```python
from build123d import *

# Parameters (mm, degrees)
SKETCH1_W               = 52
SKETCH1_H               = 46
SKETCH1_R               = 1.15
SKETCH1_R_2             = 11.5
SKETCH1_W_2             = 4.3
SKETCH1_H_2             = 18
BOSS_EXTRUDE1_DEPTH     = 4
BOSS_EXTRUDE2_DEPTH     = 4
BOSS_EXTRUDE3_DEPTH     = 44
CHAMFER1_SIZE           = 25
CUT_EXTRUDE1_DEPTH      = 70.491006612
CUT_EXTRUDE1_DEPTH_BACK = 70.491006612
SKETCH4_R               = 1.15
FILLET1_R               = 5
FILLET2_R               = 1


with BuildPart() as part:
    # Sketch1 → Boss-Extrude1 (new body)
    # profile 1 of 4: a face of its own
    with BuildSketch(Plane.XY):
        with Locations((0, -2)):
            Rectangle(SKETCH1_W, SKETCH1_H)
        with Locations((15.5, 15.5)):
            Circle(SKETCH1_R, mode=Mode.SUBTRACT)
        with Locations((15.5, -15.5)):
            Circle(SKETCH1_R, mode=Mode.SUBTRACT)
        with Locations((-15.5, -15.5)):
            Circle(SKETCH1_R, mode=Mode.SUBTRACT)
        with Locations((-15.5, 15.5)):
            Circle(SKETCH1_R, mode=Mode.SUBTRACT)
        Circle(SKETCH1_R_2, mode=Mode.SUBTRACT)
    # profile 2 of 4: a face of its own
    with BuildSketch(Plane.XY):
        with Locations((-13.488188518, -34)):
            Rectangle(SKETCH1_W_2, SKETCH1_H_2)
    # profile 3 of 4: a face of its own
    with BuildSketch(Plane.XY):
        with Locations((13.488188518, -34)):
            Rectangle(SKETCH1_W_2, SKETCH1_H_2)
    # profile 4 of 4: a face of its own
    with BuildSketch(Plane.XY):
        Polygon((3.5, -26), (4.5, -25), (-4.5, -25), (-3.5, -26), align=None)
    extrude(amount=BOSS_EXTRUDE1_DEPTH)

    # Sketch2 → Boss-Extrude2 (add)
    with BuildSketch(Plane.XY):
        Polygon((26, 21), (22, 21), (22, -17), (18, -21), (-18, -21), (-22, -17), (-22, 21), (-26, 21), (-26, -25), (-15.638188518, -25), (-15.638188518, -43), (-11.338188518, -43), (-11.338188518, -25), (-4.5, -25), (-3.5, -26), (3.5, -26), (4.5, -25), (11.338188518, -25), (11.338188518, -43), (15.638188518, -43), (15.638188518, -25), (26, -25), align=None)
    extrude(amount=-BOSS_EXTRUDE2_DEPTH)

    # Sketch3 → Boss-Extrude3 (add)
    with BuildSketch(Plane(origin=(0, 0, -4), x_dir=(-1, 0, 0), z_dir=(0, 0, -1))):
        Polygon((-26, -25), (-26, -17), (-22, -17), (-18, -21), (18, -21), (22, -17), (26, -17), (26, -25), (15.638188518, -25), (15.638188518, -43), (11.338188518, -43), (11.338188518, -25), (4.5, -25), (3.5, -26), (-3.5, -26), (-4.5, -25), (-11.338188518, -25), (-11.338188518, -43), (-15.638188518, -43), (-15.638188518, -25), align=None)
    extrude(amount=BOSS_EXTRUDE3_DEPTH)

    # Chamfer1
    chamfer1_edges = [part.edges().sort_by_distance(p)[0] for p in [
        (-24, -17, -4),
        (24, -17, -4),
    ]]
    chamfer(chamfer1_edges, length=CHAMFER1_SIZE)

    # Sketch4 → Cut-Extrude1 (cut, two sides: drawn at the far end of the back side and taken through both)
    with BuildSketch(Plane(origin=(0, 0, 0), x_dir=(0, 0, -1), z_dir=(1, 0, 0)).offset(-CUT_EXTRUDE1_DEPTH_BACK)):
        with Locations(Location((34, -35, 0), (0, 0, 270))):
            Circle(SKETCH4_R)
        with Locations(Location((12, -35, 0), (0, 0, 270))):
            Circle(SKETCH4_R)
    extrude(amount=CUT_EXTRUDE1_DEPTH + CUT_EXTRUDE1_DEPTH_BACK, mode=Mode.SUBTRACT)

    # Fillet1
    fillet1_edges = [part.edges().sort_by_distance(p)[0] for p in [
        (15.638188518, -25, -22),
        (-15.638188518, -25, -22),
    ]]
    fillet(fillet1_edges, radius=FILLET1_R)

    # Fillet2
    # the kernel refuses this fillet: 1 mm, written as the material it adds along each edge
    with BuildSketch(Plane(origin=(-22, -17, -29), x_dir=(0, 0.7071067811865475, 0.7071067811865475), z_dir=(-1, 0, 0))) as fillet2_piece_1_section:
        with BuildLine():
            CenterArc((FILLET2_R * 0.414213562373, FILLET2_R), FILLET2_R, 225, 45)
            Line((-FILLET2_R * 0.292893218813, FILLET2_R * 0.292893218813), (0, 0))
            Line((0, 0), (FILLET2_R * 0.414213562373, 0))
        make_face()
    fillet2_piece_1 = extrude(amount=4, mode=Mode.PRIVATE)
    fillet2_piece_1 = split(fillet2_piece_1, bisect_by=Plane(origin=(-22.109509858, -16.890490142, -28.87205582), z_dir=(0.7071067811865658, 0.7071067811865294, 0)), keep=Keep.TOP, mode=Mode.PRIVATE)
    add(fillet2_piece_1)
    with BuildSketch(Plane(origin=(-22, -17, -29), x_dir=(0, 0.7071067811865475, 0.7071067811865475), z_dir=(-1, 0, 0))) as fillet2_piece_2_section:
        with BuildLine():
            CenterArc((FILLET2_R * 0.414213562373, FILLET2_R), FILLET2_R, 225, 45)
            Line((-FILLET2_R * 0.292893218813, FILLET2_R * 0.292893218813), (0, 0))
            Line((0, 0), (FILLET2_R * 0.414213562373, 0))
        make_face()
    fillet2_piece_2 = extrude(amount=4, mode=Mode.PRIVATE)
    fillet2_piece_2 = split(fillet2_piece_2, bisect_by=Plane(origin=(-23.045900005, -15.954099995, -29.028101444), z_dir=(-0.7071067811865658, -0.7071067811865294, 0)), keep=Keep.TOP, mode=Mode.PRIVATE)
    add(fillet2_piece_2)
    with BuildSketch(Plane(origin=(-22, 8, -4), x_dir=(0, 1, 0), z_dir=(-1, 0, 0))) as fillet2_piece_3:
        with BuildLine():
            CenterArc((FILLET2_R * 0.414213562373, FILLET2_R), FILLET2_R, 225, 45)
            Line((-FILLET2_R * 0.292893218813, FILLET2_R * 0.292893218813), (0, 0))
            Line((0, 0), (FILLET2_R * 0.414213562373, 0))
        make_face()
    extrude(amount=4)
    with BuildSketch(Plane(origin=(26, -17, -29), x_dir=(0, 0, -1), z_dir=(-1, 0, 0))) as fillet2_piece_4_section:
        with BuildLine():
            CenterArc((FILLET2_R * 0.414213562373, -FILLET2_R), FILLET2_R, 90, 45)
            Line((-FILLET2_R * 0.292893218813, -FILLET2_R * 0.292893218813), (0, 0))
            Line((0, 0), (FILLET2_R * 0.414213562373, 0))
        make_face()
    fillet2_piece_4 = extrude(amount=4, mode=Mode.PRIVATE)
    fillet2_piece_4 = split(fillet2_piece_4, bisect_by=Plane(origin=(23.045900005, -15.954099995, -29.028101444), z_dir=(0.7071067811865454, -0.7071067811865498, 0)), keep=Keep.TOP, mode=Mode.PRIVATE)
    add(fillet2_piece_4)
    with BuildSketch(Plane(origin=(26, -17, -29), x_dir=(0, 0, -1), z_dir=(-1, 0, 0))) as fillet2_piece_5_section:
        with BuildLine():
            CenterArc((FILLET2_R * 0.414213562373, -FILLET2_R), FILLET2_R, 90, 45)
            Line((-FILLET2_R * 0.292893218813, -FILLET2_R * 0.292893218813), (0, 0))
            Line((0, 0), (FILLET2_R * 0.414213562373, 0))
        make_face()
    fillet2_piece_5 = extrude(amount=4, mode=Mode.PRIVATE)
    fillet2_piece_5 = split(fillet2_piece_5, bisect_by=Plane(origin=(22.109509858, -16.890490142, -28.87205582), z_dir=(-0.7071067811865454, 0.7071067811865498, 0)), keep=Keep.TOP, mode=Mode.PRIVATE)
    add(fillet2_piece_5)
    with BuildSketch(Plane(origin=(26, 8, -4), x_dir=(0, -0.7071067811865475, -0.7071067811865475), z_dir=(-1, 0, 0))) as fillet2_piece_6:
        with BuildLine():
            CenterArc((FILLET2_R * 0.414213562373, -FILLET2_R), FILLET2_R, 90, 45)
            Line((-FILLET2_R * 0.292893218813, -FILLET2_R * 0.292893218813), (0, 0))
            Line((0, 0), (FILLET2_R * 0.414213562373, 0))
        make_face()
    extrude(amount=4)
    # the kernel refuses this fillet: 1 mm, written as the material it takes off along each edge
    with BuildSketch(Plane(origin=(-19.5, -17, -48), x_dir=(0, -1, 0), z_dir=(-1, 0, 0)), Plane(origin=(-19.5, 21, -4), x_dir=(0, -1, 0), z_dir=(-1, 0, 0)), Plane(origin=(28.5, 21, -4), x_dir=(0, -1, 0), z_dir=(-1, 0, 0))) as fillet2_2_piece_1:
        with BuildLine():
            CenterArc((FILLET2_R, FILLET2_R), FILLET2_R, 180, 90)
            Line((0, FILLET2_R), (0, 0))
            Line((0, 0), (FILLET2_R, 0))
        make_face()
    extrude(amount=9, mode=Mode.SUBTRACT)
    with BuildSketch(Plane(origin=(28.5, -17, -48), x_dir=(0, 0, 1), z_dir=(-1, 0, 0))) as fillet2_2_piece_2:
        with BuildLine():
            CenterArc((FILLET2_R, -FILLET2_R), FILLET2_R, 90, 90)
            Line((0, -FILLET2_R), (0, 0))
            Line((0, 0), (FILLET2_R, 0))
        make_face()
    extrude(amount=9, mode=Mode.SUBTRACT)
    with BuildSketch(Plane(origin=(26, -25, 6.5), x_dir=(0, 1, 0), z_dir=(0, 0, -1)), Plane(origin=(-15.638188518, -43, 6.5), x_dir=(1, 0, 0), z_dir=(0, 0, -1))) as fillet2_2_piece_3:
        with BuildLine():
            CenterArc((FILLET2_R, -FILLET2_R), FILLET2_R, 90, 90)
            Line((0, -FILLET2_R), (0, 0))
            Line((0, 0), (FILLET2_R, 0))
        make_face()
    extrude(amount=57, mode=Mode.SUBTRACT)
    with BuildSketch(Plane(origin=(15.638188518, -43, 6.5), x_dir=(-1, 0, 0), z_dir=(0, 0, -1)), Plane(origin=(-26, -25, -50.5), x_dir=(1, 0, 0), z_dir=(0, 0, 1))) as fillet2_2_piece_4:
        with BuildLine():
            CenterArc((FILLET2_R, FILLET2_R), FILLET2_R, 180, 90)
            Line((0, FILLET2_R), (0, 0))
            Line((0, 0), (FILLET2_R, 0))
        make_face()
    extrude(amount=57, mode=Mode.SUBTRACT)


solid = part.part
```
Geometry: final body of the model. Coordinates: model frame, mm. A direction names the side the tool comes from. Round coordinates to 2 decimals unless told otherwise and drop trailing zeros. Write each loop counter-clockwise with the first axis right and the second up, starting at its lowest first coordinate (ties: lowest second). Pieces come first, ordered by that corner, then holes. Notation, with made-up numbers: (35.25, 66.5) -> (64.25, 66.5) arc R26 cw to (64.25, 90.5) -> close; hole circle Ø6 at (-36.75, 87). An arc over 180 degrees is marked (long way). Return JSON: item names as keys, results as strings.
Q1. Section D-D on y = 15.5. Return the cut outline in (x, z).
From the geometry:
{"outline": "(-26, -4) -> (-22, -4) -> (-22, 0) -> (-16.65, 0) -> (-16.65, 4) -> (-26, 4) -> close; (-14.35, 0) -> (14.35, 0) -> (14.35, 4) -> (-14.35, 4) -> close; (16.65, 0) -> (22, 0) -> (22, -4) -> (26, -4) -> (26, 4) -> (16.65, 4) -> close"}
Q2. Section A-A on z = -34. Give the number of separate pieces and of enclosed holes in the cut face, and give its area (3 significant figures).
From the geometry:
{"separate pieces": "3", "enclosed holes": "0", "area": "409 mm2"}
Q3. Section C-C on x = 0. Return the cut outline in (y, z), and give its area (3 significant figures).
From the geometry:
{"outline": "(-26, -48) -> (-21, -48) -> (-21, 0) -> (-11.5, 0) -> (-11.5, 4) -> (-26, 4) -> close; (11.5, 0) -> (21, 0) -> (21, 4) -> (11.5, 4) -> close", "area": "336 mm2"}
Q4. Set-up query: faces 1 (the flat face through (22, -5, -8)), 2 (the flat face through (-24, -17, -38)), 3 (the flat face through (8, -25, -22)). Return all of +Z, -Z, +X, -X, +Y, -Y with unobstructed straight access to the full face (end or side cutting, diameter ignored); none if empty.
From the geometry:
{"face 1": "-Z, +Y", "face 2": "-Z, +X, -X, +Y", "face 3": "+Z, -Z, -Y"}
Q5. Section B-B on y = -38.5. Return the cut outline in (x, z), and give its area (3 significant figures).
From the geometry:
{"outline": "(-15.64, -48) -> (-11.34, -48) -> (-11.34, 4) -> (-15.64, 4) -> close; (11.34, -48) -> (15.64, -48) -> (15.64, 4) -> (11.34, 4) -> close", "area": "447 mm2"}
Q6. Ray query, line 1 (X direction, y = -18, z = -23.5); line 2 (X direction, y = -13, z = -18); line 3 (Z direction, x = -13.5, y = 13.5). Return the intervals inside material, ascending.
From the geometry:
{"line 1": "-26 to -21, 21 to 26", "line 2": "-26 to -22, 22 to 26", "line 3": "0 to 4"}
Q7. Mould query, pull axis X, two halves, no side actions, for faces 4 (the flat face through (0, -21, -24)), 5 (the flat face through (-23, -25, -22)), 6 (the flat face through (-10, 10, 0)), 7 (the flat face through (15.638, -36, -22)). Classes: +X half, -X half, draft (parallel to the pull), parting line (faces both ways), or undercut.
From the geometry:
{"face 4": "undercut", "face 5": "draft", "face 6": "undercut", "face 7": "+X half"}
Q8. First-contact query: pin 1 Ø10 at (x, y) = (-14.5, 2) entering from -Z; pin 2 Ø6 at (y, z) = (-35, -18) entering from -X; pin 3 Ø3 at (x, z) = (-9, -38) entering from +Y. Flat tips, straight axial feed; report the tip coordinate or a pass-through.
From the geometry:
{"pin 1": "z = 0", "pin 2": "x = -15.64", "pin 3": "y = -21"}
